Autodesk Inventor part; units mm, degrees
ref_plane "Work Plane1" through (0, 0, 50) normal (0, 0, 1) x (1, 0, 0)
ref_plane "YZ Plane" through (0, 0, 0) normal (1, 0, 0) x (0, 1, 0)
ref_plane "XZ Plane" through (0, 0, 0) normal (0, 1, 0) x (-1, 0, 0)
sketch "Sketch1" plane through (0, 0, 0) normal (0, 0, 1) x (1, 0, 0)
  circle A0 centre (0, 0) radius 3.5
  dimension "d0" = 7
extrude "Extrusion1" add sketch "Sketch1" along normal blind 100
ref_plane "Work Plane1" through (0, 0, 50) normal (0, 0, 1) x (1, 0, 0)
sketch "Sketch2" plane through (0, 0, 50) normal (0, 0, 1) x (1, 0, 0)
  circle A0 centre (0, 0) radius 3.5
  line L0 (-2, 2.8723) -> (-2, 4.8723)
  line L1 (-2, 4.8723) -> (2, 4.8723)
  line L2 (2, 4.8723) -> (2, 2.8723)
  circle A1 centre (0, 0) radius 3.5
  arc A2 (2, 2.8723) -> (-2, 2.8723) centre (0, 0) ccw
  circle A3 centre (0, 0) radius 3.5
  point P0 (0, 4.8723)
  dimension "d4" = 4
  dimension "d5" = 2
extrude "Extrusion2" add sketch "Sketch2" along normal mid plane 50 contours A0 L0 L1 L2
properties part number "shaft2"
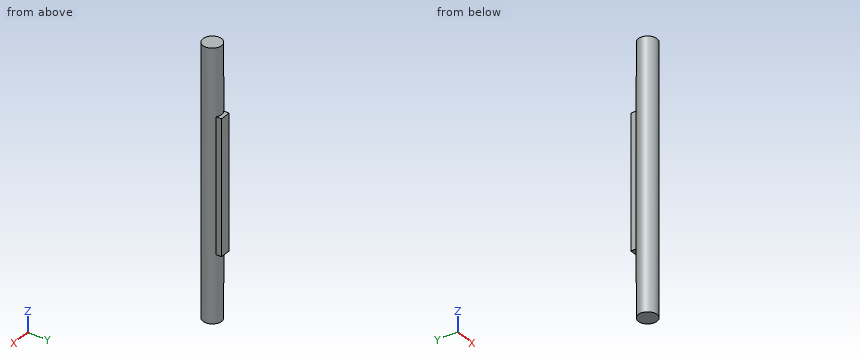
Could you check a few things on this model? Use its own coordinates, in mm. Give positions to 0.01 mm unless a question says otherwise; leave off trailing zeros. Write each loop counter-clockwise with the first axis right and the second up, starting at its lowest first coordinate (ties: lowest second). Pieces come first, ordered by that corner, then holes. Notation, with made-up numbers: (21, 62.25) - (28, 62.25) arc R23 ccw to (28, 86.25) - close; hole circle Ø2 at (76, 7.5). An arc over 180 degrees is marked (long way). Use CSV: the item, a comma, the result in double quotes. Start each with the question number.
Item 1: I want a section at A-A, the plane x = 0. Please give me the cut outline in (y, z).
Item 2: I want a section at D-D, the plane z = 86.5. Please give me the cut outline in (x, y), then the cut area to 3 significant figures.
Item 3: I want a section at B-B, the plane z = 56. Please give me the cut outline in (x, y), then the cut area to 3 significant figures.
Item 4: I want a section at C-C, the plane y = -2.5. Please give me the cut outline in (x, z), then the cut area to 3 significant figures.
Item 5: If I drill on line 1 along Z through (x, y) = (-1, 3.75); line 2 along X through (y, z) = (0.25, 16.5); line 3 along Y through (x, z) = (1, 86), over which ranges is the centre line in solid material (lowest first)?
Item 6: I'm going to push flat-ended pins straight in: pin 1 (1 mm diameter, centred on y = 4, z = 53, fed in from +X); pin 2 (0.6 mm diameter, centred on y = 4, z = 53, fed in from -X); pin 3 (2 mm diameter, centred on y = 2.5, z = 28.5, fed in from -X). Where does each tip first touch, or does it pass through?
Findings:
1,outline,"(-3.5, 0) - (3.5, 0) - (3.5, 25) - (4.87, 25) - (4.87, 75) - (3.5, 75) - (3.5, 100) - (-3.5, 100) - close"
2,outline,"circle Ø7 at (0, 0)"
2,area,"38.5 mm2"
3,outline,"(-2, 2.87) arc R3.5 ccw (long way) to (2, 2.87) - (2, 4.87) - (-2, 4.87) - close"
3,area,"44.8 mm2"
4,outline,"(-2.45, 0) - (2.45, 0) - (2.45, 100) - (-2.45, 100) - close"
4,area,"490 mm2"
5,line 1,"z = 25 to 75"
5,line 2,"x = -3.49 to 3.49"
5,line 3,"y = -3.35 to 3.35"
6,pin 1,"stops at x = 2"
6,pin 2,"stops at x = -2"
6,pin 3,"stops at x = -3.16"
